Source: CAD feature listing. Evaluate the final solid. Frame: model axes, mm. Face numbers are marked on the shaded views. A direction names the side the tool comes from. Round coordinates to 2 decimals unless told otherwise and drop trailing zeros. Write each loop counter-clockwise with the first axis right and the second up, starting at its lowest first coordinate (ties: lowest second). Pieces come first, ordered by that corner, then holes. Notation, with made-up numbers: M 17,75.25 L 63,75.25 A24 ccw 63,87.25 Z; hole C 32.25,25 d2. An arc over 180 degrees is marked long. Put each result on its own line as item: value. Start each with the question number.
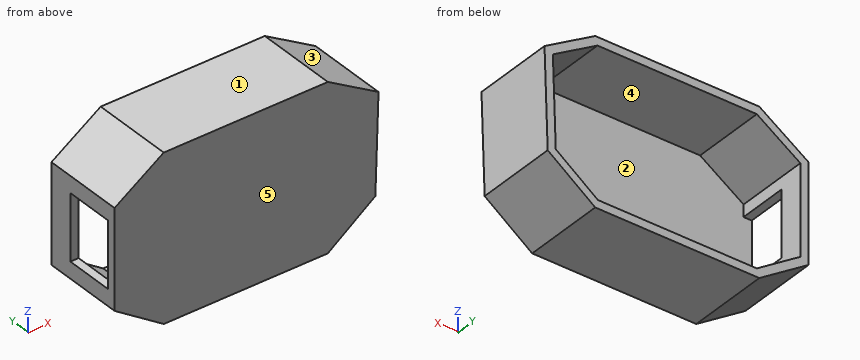
```python
from build123d import *

# Parameters (mm, degrees)
DODANIE_WYCI_GNI_CIE2_DEPTH = 50
SKORUPA2_T                  = -5
WYTNIJ_WYCI_GNI_CIE1_REACH  = 162.907
SZKIC2_W                    = 40
SZKIC2_H                    = 30


with BuildPart() as part:
    # Szkic1 → Dodanie-wyciągnięcie2 (new body)
    with BuildSketch(Plane(origin=(0, 0, 0), x_dir=(1, 0, 0), z_dir=(0, 1, 0))):
        Polygon((-60, 40), (40, 40), (68.970961298, 18.536463444), (70.906962059, -41.432294264), (40, -60), (-60, -60), (-90, -40), (-90, 20), align=None)
    extrude(amount=DODANIE_WYCI_GNI_CIE2_DEPTH)

    # Skorupa2
    skorupa2_openings = [part.faces().sort_by_distance(p)[0] for p in [
        (-10.01525958, 50, 10.361978853),
    ]]
    offset(amount=SKORUPA2_T, openings=skorupa2_openings, kind=Kind.INTERSECTION)

    # Szkic2 → Wytnij-wyciągnięcie1 (cut, up to next)
    with BuildSketch(Plane.ZY.offset(90), mode=Mode.PRIVATE) as wytnij_wyci_gni_cie1_sk1:
        with Locations((10, 20)):
            Rectangle(SZKIC2_W, SZKIC2_H)
    wytnij_wyci_gni_cie1_tool1 = extrude(wytnij_wyci_gni_cie1_sk1.sketch, amount=-WYTNIJ_WYCI_GNI_CIE1_REACH, mode=Mode.PRIVATE) & part.part
    add(wytnij_wyci_gni_cie1_tool1.solids().sort_by_distance((-90, 20, 10))[0], mode=Mode.SUBTRACT)


solid = part.part
```
(1) Pull-direction query (X, two-part tool) for the marked faces 1, 2 and 3; classes: +X half, -X half, draft (parallel to the pull), parting line (faces both ways), or undercut.
(2) Section query A-A (z = 1). Return loops of the section in (x, y).
(3) Section query D-D (x = -14.5). Return loops of the section in (y, z), and give its area (3 significant figures).
(4) Section query B-B (y = 18.5). Return loops of the section in (x, z), and give its area (3 significant figures).
(5) Section query C-C (y = 46.5). Return loops of the section in (x, z).
(6) Ray query, line 1 along Z through (x, y) = (-8.5, 30); line 2 along Y through (x, z) = (-75.5, -17); line 3 along X through (y, z) = (14.5, 42.5). Return the intervals inside material, ascending.
(7) Contact query for flat-ended pins moving along their axis: P1, Ø4, axis at y = 42.5, z = -19.5, coming from the +X side; P2, Ø5, axis at y = 38.5, z = 20, coming from the +X side; P3, Ø4, axis at y = 26, z = -22.5, coming from the -X side. Output: stop coordinate, or through.
(8) Access query for the marked faces 4 and 5. Directions: +Z, -Z, +X, -X, +Y, -Y. A direction counts if a zero-diameter tool reaches every point of the face in a straight line with its end or side. Return the directions, or none.
Entries:
1. face 1: draft
1. face 2: undercut
1. face 3: +X half
2. outline: M -90,0 L 69.6,0 L 69.6,50 L 64.6,50 L 64.6,5 L -90,5 Z; M -90,35 L -85,35 L -85,50 L -90,50 Z
3. outline: M 0,-40 L 50,-40 L 50,-35 L 5,-35 L 5,55 L 50,55 L 50,60 L 0,60 Z
3. area: 950 mm2
4. outline: M -90,-20 L -60,-40 L 40,-40 L 68.97,-18.54 L 70.91,41.43 L 40,60 L -60,60 L -90,40 L -90,30 L -85,30 L -85,37.32 L -58.49,55 L 38.61,55 L 65.81,38.66 L 64.05,-15.96 L 38.35,-35 L -58.49,-35 L -85,-17.32 L -85,-10 L -90,-10 Z
4. area: 2,040 mm2
5. outline: M -90,-20 L -60,-40 L 40,-40 L 68.97,-18.54 L 70.91,41.43 L 40,60 L -60,60 L -90,40 Z; hole M -85,-17.32 L -58.49,-35 L 38.35,-35 L 64.05,-15.96 L 65.81,38.66 L 38.61,55 L -58.49,55 L -85,37.32 Z
6. line 1: -40 to -35, 55 to 60
6. line 2: 0 to 5
6. line 3: -86.25 to -77.24, 59.42 to 69.13
7. P1: x = 69
7. P2: x = 70.3
7. P3: x = -89.25
8. face 4: +Y
8. face 5: +Z, -Z, +X, -X, -Y
